from build123d import *

# Parameters (mm, degrees)
F1_DEPTH = 101.6
F2_T     = -6.35
F3_W     = 63.5
F3_H     = 3.175
F4_DEPTH = 95.25


with BuildPart() as f1:
    # F0 (on Front) → F1 (new body)
    with BuildSketch(Plane.XZ):
        with BuildLine():
            Line((34.29, 76.2), (-34.29, 76.2))
            ThreePointArc((-34.29, 76.2), (-36.984077, 75.084077), (-38.1, 72.39))
            Line((-38.1, 72.39), (-38.1, -72.39))
            ThreePointArc((-38.1, -72.39), (-36.984077, -75.084077), (-34.29, -76.2))
            Line((-34.29, -76.2), (34.29, -76.2))
            ThreePointArc((34.29, -76.2), (36.984077, -75.084077), (38.1, -72.39))
            Line((38.1, -72.39), (38.1, 72.39))
            ThreePointArc((38.1, 72.39), (36.984077, 75.084077), (34.29, 76.2))
        make_face()
    extrude(amount=F1_DEPTH)

    # F2
    f2_openings = [f1.faces().sort_by_distance(p)[0] for p in [
        (0, -101.6, 0),
    ]]
    offset(amount=F2_T, openings=f2_openings)

    # F3 (on face) → F4 (join)
    with BuildSketch(Plane.XZ.offset(6.35)):
        with Locations((0, 12.657333)):
            Rectangle(F3_W, F3_H)
    extrude(amount=F4_DEPTH)


solid = f1.part
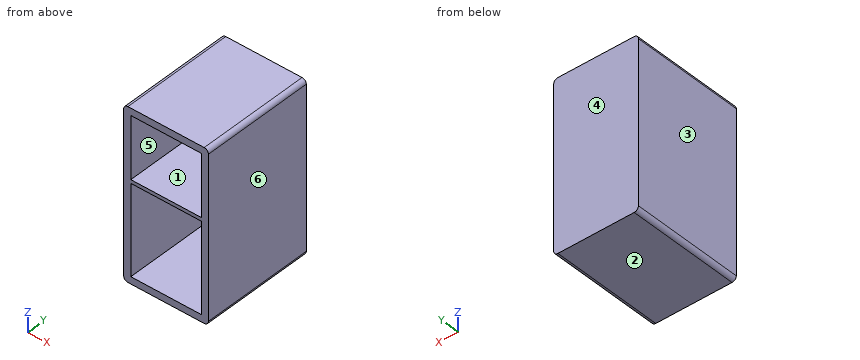
Design review of the part built by this model. Coordinates are the model's own, in mm. Face numbers are marked on the shaded views. A direction names the side the tool comes from. Coordinates: 2 decimals unless noted, no trailing zeros. Loops run counter-clockwise (first coordinate to the right, second up) from the corner with the lowest first, then second, coordinate; pieces in that order, holes last. Notation, with made-up numbers: M 70.5,-29.75 L 80.5,-29.75 A18 cw 80.5,-7.75 Z; hole C 74.5,24 d11. An arc over 180 degrees is marked long. Use one line per item in the form item = value.
(1) Consider section C-C (x = -17). Write out the cut boundary in (y, z).
Return value:
outline = M -101.6,-76.2 L 0,-76.2 L 0,76.2 L -101.6,76.2 L -101.6,69.85 L -6.35,69.85 L -6.35,14.24 L -101.6,14.24 L -101.6,11.07 L -6.35,11.07 L -6.35,-69.85 L -101.6,-69.85 Z
(2) Clearance check with flat-ended pins moving along their axes: P1, Ø6, axis at x = 20, z = 37.5, coming from the +Y side; P2, Ø3, axis at x = 14, z = -37, coming from the -Y side. State where each tip first meets the part, or that it passes through.
Return value:
P1 = 0
P2 = -6.35
(3) For the marked faces 1 and 2, list the 3-axis set-ups (+Z, -Z, +X, -X, +Y, -Y) from which the entire face can be reached by the end or side of a thin tool; tool diameter is ignored.
Return value:
face_1 = -Y
face_2 = -Z, +X, -X, +Y, -Y
(4) For line 1 along Z through (x, y) = (8, -42); line 2 along X through (y, z) = (-32.5, -33.5), list the stretches that pass through material, from the lowest coordinate up. Write a range as from..to.
Return value:
line_1 = -76.2..-69.85, 11.07..14.24, 69.85..76.2
line_2 = -38.1..-31.75, 31.75..38.1
(5) Draft analysis for pull direction X (two halves, no side actions). For the marked faces 3, 4, 5 and 6, state which applies: pulls with the +X half, pulls with the -X half, needs draft (parallel to the pull), parting line crosses it, or undercut.
Return value:
face_3 = pulls with the -X half
face_4 = needs draft
face_5 = undercut
face_6 = pulls with the +X half
(6) Consider section B-B (z = -19). Write out the cut boundary in (x, y).
Return value:
outline = M -38.1,-101.6 L -31.75,-101.6 L -31.75,-6.35 L 31.75,-6.35 L 31.75,-101.6 L 38.1,-101.6 L 38.1,0 L -38.1,0 Z
(7) Consider section A-A (y = -45). Write out the cut boundary in (x, z).
Return value:
outline = M -38.1,-72.39 A3.81 ccw -34.29,-76.2 L 34.29,-76.2 A3.81 ccw 38.1,-72.39 L 38.1,72.39 A3.81 ccw 34.29,76.2 L -34.29,76.2 A3.81 ccw -38.1,72.39 Z; hole M -31.75,-69.85 L 31.75,-69.85 L 31.75,11.07 L -31.75,11.07 Z; hole M -31.75,14.24 L 31.75,14.24 L 31.75,69.85 L -31.75,69.85 Z
